Could you check a few things on this model? Use its own coordinates, in mm. A direction names the side the tool comes from. Round coordinates to 2 decimals unless told otherwise and drop trailing zeros. Write each loop counter-clockwise with the first axis right and the second up, starting at its lowest first coordinate (ties: lowest second). Pieces come first, ordered by that corner, then holes. Notation, with made-up numbers: (40.25, -8.75) - (88.25, -8.75) arc R17 cw to (88.25, 0.25) - close; hole circle Ø8 at (11.25, -12). An arc over 180 degrees is marked (long way). Write each question's results on one line, items separated by ' | '. Start each with the question number.
(1) On a 3-axis mill with a long thin cutter (end or side, diameter ignored), from which of +Z, -Z, +X, -X, +Y, -Y can I reach the whole of each face in a straight line? I mean faces 4 (the cylindrical face through (25.67, 24.24, -33.48)), 5 (the cylindrical face through (-37.208, 3.571, -40.577)), 6 (the cylindrical face through (-2.94, 8.16, 74.76)). Say none if no direction works.
(2) For P1, Ø1, axis at x = 49, z = 7, coming from the -Y side; P2, Ø2, axis at y = 15, z = -59, coming from the +X side; P3, Ø5, axis at y = 20.5, z = 49.5, coming from the +X side, each with a flat end and sliding along its axis, tell me the tip position at first contact or that it passes through.
(3) Please list where these lines run through material, in increasing order: line 1 (X direction, y = 4, z = 0); line 2 (Y direction, x = -69.5, z = 23); line 3 (Z direction, x = -12.5, y = 11). Write a range as [from, to].
(4) Thinking about a two-plate mould opening in X: for faces 1 (the cylindrical face through (65.09, 8.16, -38.4)), 2 (the cylindrical face through (31.831, 24.703, -41.512)), 3 (the flat face through (53, 16.104, 1)), which applies, +X half, -X half, draft (parallel to the pull), parting line (faces both ways), or undercut?
(5) Imagine slicing it at C-C on x = 0. State how many separate pieces and enclosed holes the cut face has, then the cut area to 3 significant figures.
(6) Imagine slicing it at B-B on y = 24.5. Write out the boundary of the cut face in (x, z).
```python
from build123d import *

# Parameters (mm, degrees)
F2_SIZE = 1.5748
F3_R    = 0.508
F5_D    = 10.9474


with BuildPart() as f1:
    # F0 (on Right) → F1 (revolve)
    with BuildSketch(Plane.YZ):
        Polygon((16.1036, 80.9625), (0, 80.9625), (0, 55.0545), (5.5118, 55.0545), (5.5118, 47.625), (10.382705, 37.6555), (14.675305, 37.6555), (14.675305, 42.1894), (35.122305, 42.1894), (35.122305, 52.3113), (16.1036, 52.3113), align=None)
    revolve(axis=Axis((0, 17.561152, 0), (0, -1, 0)))

    # F2
    f2_edges = [f1.edges().sort_by_distance(p)[0] for p in [
        (0, 35.122305, -42.1894),
        (0, 35.122305, -52.3113),
        (0, 0, -55.0545),
    ]]
    chamfer(f2_edges, length=F2_SIZE)

    # F3
    f3_edges = [f1.edges().sort_by_distance(p)[0] for p in [
        (0, 14.675305, -37.6555),
        (0, 16.1036, -80.9625),
        (0, 0, -80.9625),
    ]]
    fillet(f3_edges, radius=F3_R)

    # F5 (through all)
    with Locations(Plane.XZ):
        with Locations((0, 70.1421), (60.74484, 35.07105), (60.74484, -35.07105), (0, -70.1421), (-60.74484, -35.07105), (-60.74484, 35.07105)):
            Hole(F5_D / 2)


solid = f1.part
```
Response:
1) face 4: +Y | face 5: -Y | face 6: +Y, -Y
2) P1: y = 5.51 | P2: x = 56.49 | P3: x = 22.97
3) line 1: [-80.96, -55.05], [55.05, 80.96] | line 2: [0, 16.1] | line 3: [-79.99, -35.52], [35.52, 79.99]
4) face 1: undercut | face 2: parting line | face 3: draft
5) separate pieces: 4 | enclosed holes: 0 | area: 1,170 mm²
6) outline: circle Ø104.62 at (0, 0); hole circle Ø84.38 at (0, 0)
